Could you check a few things on this model? Use its own coordinates, in mm. Face numbers are marked on the shaded views. A direction names the side the tool comes from. Coordinates: 2 decimals unless noted, no trailing zeros. Order: outer loops, then holes, each group sorted by start corner. A loop starts at its lowest first (then second) coordinate and runs counter-clockwise, first axis right, second up. Notation, with made-up numbers: (26.5, -25) -> (83.5, -25) arc R30 ccw to (83.5, 4) -> close; hole circle Ø5 at (81.5, 52). An arc over 180 degrees is marked (long way). Return JSON: item names as keys, results as strings. Group by question number.
from build123d import *

# Parameters (mm, degrees)
EXTRUDE1_DEPTH                         = 25.4
EXTRUDE1_DEPTH_BACK                    = 50.8
SKETCH2_W                              = 119.38
SKETCH2_H                              = 22.225
EXTRUDE2_DEPTH                         = 3.175
SKETCH3_W                              = 3.175
SKETCH3_H                              = 22.225
EXTRUDE3_DEPTH                         = 19.05
TAP_DRILL_FOR_1_2_TAP1_D               = 11.50874
TAP_DRILL_FOR_1_2_TAP1_DEPTH           = 6.35
TAP_DRILL_FOR_1_2_TAP1_TIP             = 3.45757432
TAP_DRILL_FOR_1_2_TAP1_ON_FACE_2_D     = 11.50874
TAP_DRILL_FOR_1_2_TAP1_ON_FACE_2_DEPTH = 6.35
TAP_DRILL_FOR_1_2_TAP1_ON_FACE_2_TIP   = 3.45757432
F_8_CLEARANCE_HOLE1_D                  = 4.4958
F_8_CLEARANCE_HOLE1_DEPTH              = 6.35
F_8_CLEARANCE_HOLE1_TIP                = 1.350674586
F_8_CLEARANCE_HOLE1_ON_FACE_2_D        = 4.4958
F_8_CLEARANCE_HOLE1_ON_FACE_2_DEPTH    = 6.35
F_8_CLEARANCE_HOLE1_ON_FACE_2_TIP      = 1.350674586
FILLET1_R                              = 6.35
FILLET3_R                              = 3.175
SKETCH7_W                              = 81.28
SKETCH7_H                              = 3.175
EXTRUDE4_DEPTH                         = 25.4
FILLET4_R                              = 6.35
F_6_CLEARANCE_HOLE1_D                  = 3.7973
F_6_CLEARANCE_HOLE1_DEPTH              = 9.652
F_6_CLEARANCE_HOLE1_TIP                = 1.140824014
SKETCH8_W                              = 66.338719692
SKETCH8_H                              = 61.141500313
CUT_EXTRUDE1_DEPTH                     = 57.15


with BuildPart() as part:
    # Sketch1 → Extrude1 (new body, two sides)
    with BuildSketch(Plane(origin=(0, 0, 0), x_dir=(1, 0, 0), z_dir=(0, 1, 0))) as extrude1_sk:
        with BuildLine():
            Line((15.24, -11.1125), (-15.24, -11.1125))
            ThreePointArc((-15.24, -11.1125), (-19.730128061, -9.252628061), (-21.59, -4.7625))
            Line((-21.59, -4.7625), (-21.59, 4.7625))
            ThreePointArc((-21.59, 4.7625), (-19.730128061, 9.252628061), (-15.24, 11.1125))
            Line((-15.24, 11.1125), (15.24, 11.1125))
            ThreePointArc((15.24, 11.1125), (19.730128061, 9.252628061), (21.59, 4.7625))
            Line((21.59, 4.7625), (21.59, -4.7625))
            ThreePointArc((21.59, -4.7625), (19.730128061, -9.252628061), (15.24, -11.1125))
        make_face()
        with BuildLine():
            Line((-15.24, -7.9375), (-5.715, -7.9375))
            ThreePointArc((-5.715, -7.9375), (-3.46993597, -7.00756403), (-2.54, -4.7625))
            Line((-2.54, -4.7625), (-2.54, 4.7625))
            ThreePointArc((-2.54, 4.7625), (-3.46993597, 7.00756403), (-5.715, 7.9375))
            Line((-5.715, 7.9375), (-15.24, 7.9375))
            ThreePointArc((-15.24, 7.9375), (-17.48506403, 7.00756403), (-18.415, 4.7625))
            Line((-18.415, 4.7625), (-18.415, -4.7625))
            ThreePointArc((-18.415, -4.7625), (-17.48506403, -7.00756403), (-15.24, -7.9375))
        make_face(mode=Mode.SUBTRACT)
        with BuildLine():
            Line((15.24, 7.9375), (5.715, 7.9375))
            ThreePointArc((5.715, 7.9375), (3.46993597, 7.00756403), (2.54, 4.7625))
            Line((2.54, 4.7625), (2.54, -4.7625))
            ThreePointArc((2.54, -4.7625), (3.46993597, -7.00756403), (5.715, -7.9375))
            Line((5.715, -7.9375), (15.24, -7.9375))
            ThreePointArc((15.24, -7.9375), (17.48506403, -7.00756403), (18.415, -4.7625))
            Line((18.415, -4.7625), (18.415, 4.7625))
            ThreePointArc((18.415, 4.7625), (17.48506403, 7.00756403), (15.24, 7.9375))
        make_face(mode=Mode.SUBTRACT)
    extrude(amount=EXTRUDE1_DEPTH)
    extrude(extrude1_sk.sketch, amount=-EXTRUDE1_DEPTH_BACK)

    # Sketch2 → Extrude2 (add)
    with BuildSketch(Plane(origin=(0, 25.4, 0), x_dir=(-1, 0, 0), z_dir=(0, 1, 0))):
        Rectangle(SKETCH2_W, SKETCH2_H)
    extrude(amount=EXTRUDE2_DEPTH)

    # Sketch3 → Extrude3 (add)
    with BuildSketch(Plane.XZ.offset(-25.4)):
        with Locations((-58.1025, 0)):
            Rectangle(SKETCH3_W, SKETCH3_H)
        with Locations((58.1025, 0)):
            Rectangle(SKETCH3_W, SKETCH3_H)
    extrude(amount=EXTRUDE3_DEPTH)

    # Tap Drill for 1/2 Tap1
    with Locations(Plane(origin=(-59.69, 15.875, 0), x_dir=(0, 0, -1), z_dir=(-1, 0, 0))):
        with Locations((0, 0)):
            Hole(TAP_DRILL_FOR_1_2_TAP1_D / 2, depth=TAP_DRILL_FOR_1_2_TAP1_DEPTH)
            with Locations((0, 0, -(TAP_DRILL_FOR_1_2_TAP1_DEPTH + TAP_DRILL_FOR_1_2_TAP1_TIP / 2))):  # 118° drill point
                Cone(0, TAP_DRILL_FOR_1_2_TAP1_D / 2, TAP_DRILL_FOR_1_2_TAP1_TIP, mode=Mode.SUBTRACT)

    # Tap Drill for 1/2 Tap1 on face 2
    with Locations(Plane(origin=(59.69, 15.875, 0), x_dir=(0, 0, 1), z_dir=(1, 0, 0))):
        with Locations((0, 0)):
            Hole(TAP_DRILL_FOR_1_2_TAP1_ON_FACE_2_D / 2, depth=TAP_DRILL_FOR_1_2_TAP1_ON_FACE_2_DEPTH)
            with Locations((0, 0, -(TAP_DRILL_FOR_1_2_TAP1_ON_FACE_2_DEPTH + TAP_DRILL_FOR_1_2_TAP1_ON_FACE_2_TIP / 2))):  # 118° drill point
                Cone(0, TAP_DRILL_FOR_1_2_TAP1_ON_FACE_2_D / 2, TAP_DRILL_FOR_1_2_TAP1_ON_FACE_2_TIP, mode=Mode.SUBTRACT)

    # #8 Clearance Hole1
    with Locations(Plane(origin=(-21.59, 15.875, 0), x_dir=(0, 0, -1), z_dir=(-1, 0, 0))):
        with Locations((0, 0)):
            Hole(F_8_CLEARANCE_HOLE1_D / 2, depth=F_8_CLEARANCE_HOLE1_DEPTH)
            with Locations((0, 0, -(F_8_CLEARANCE_HOLE1_DEPTH + F_8_CLEARANCE_HOLE1_TIP / 2))):  # 118° drill point
                Cone(0, F_8_CLEARANCE_HOLE1_D / 2, F_8_CLEARANCE_HOLE1_TIP, mode=Mode.SUBTRACT)

    # #8 Clearance Hole1 on face 2
    with Locations(Plane(origin=(21.59, 15.875, 0), x_dir=(0, 0, 1), z_dir=(1, 0, 0))):
        with Locations((0, 0)):
            Hole(F_8_CLEARANCE_HOLE1_ON_FACE_2_D / 2, depth=F_8_CLEARANCE_HOLE1_ON_FACE_2_DEPTH)
            with Locations((0, 0, -(F_8_CLEARANCE_HOLE1_ON_FACE_2_DEPTH + F_8_CLEARANCE_HOLE1_ON_FACE_2_TIP / 2))):  # 118° drill point
                Cone(0, F_8_CLEARANCE_HOLE1_ON_FACE_2_D / 2, F_8_CLEARANCE_HOLE1_ON_FACE_2_TIP, mode=Mode.SUBTRACT)

    # Fillet1
    fillet1_edges = [part.edges().sort_by_distance(p)[0] for p in [
        (-58.1025, 6.35, -11.1125),
        (-58.1025, 6.35, 11.1125),
        (58.1025, 6.35, 11.1125),
        (58.1025, 6.35, -11.1125),
    ]]
    fillet(fillet1_edges, radius=FILLET1_R)

    # Fillet3
    fillet3_edges = [part.edges().sort_by_distance(p)[0] for p in [
        (-56.515, 25.4, 0),
        (56.515, 25.4, 0),
    ]]
    fillet(fillet3_edges, radius=FILLET3_R)

    # Sketch7 → Extrude4 (add)
    with BuildSketch(Plane.XY.offset(11.1125)):
        with Locations((0, 26.9875)):
            Rectangle(SKETCH7_W, SKETCH7_H)
    extrude(amount=EXTRUDE4_DEPTH)

    # Fillet4
    fillet4_edges = [part.edges().sort_by_distance(p)[0] for p in [
        (-40.64, 26.9875, 11.1125),
        (40.64, 26.9875, 11.1125),
    ]]
    fillet(fillet4_edges, radius=FILLET4_R)

    # #6 Clearance Hole1
    with Locations(Plane(origin=(31.75, 28.575, 26.9875), x_dir=(0, 0, 1), z_dir=(0, 1, 0))):
        with Locations((0, 0), (0, -63.5)):
            Hole(F_6_CLEARANCE_HOLE1_D / 2, depth=F_6_CLEARANCE_HOLE1_DEPTH)
            with Locations((0, 0, -(F_6_CLEARANCE_HOLE1_DEPTH + F_6_CLEARANCE_HOLE1_TIP / 2))):  # 118° drill point
                Cone(0, F_6_CLEARANCE_HOLE1_D / 2, F_6_CLEARANCE_HOLE1_TIP, mode=Mode.SUBTRACT)

    # Sketch8 → Cut-Extrude1 (cut)
    with BuildSketch(Plane.XZ.offset(50.8)):
        with Locations((-0.031295894, -3.796156427)):
            Rectangle(SKETCH8_W, SKETCH8_H)
    extrude(amount=-CUT_EXTRUDE1_DEPTH, mode=Mode.SUBTRACT)


solid = part.part
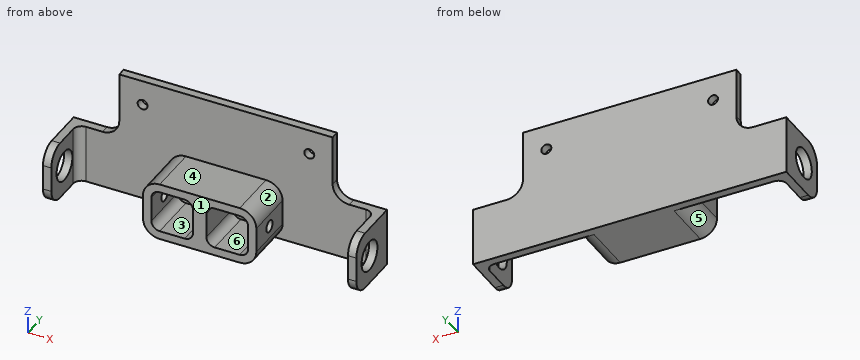
Q1. I'm going to push flat-ended pins straight in: pin 1 Ø10.5 at (x, y) = (8, 20) entering from +Z; pin 2 Ø6 at (x, z) = (39, 1) entering from -Y; pin 3 Ø1.5 at (x, y) = (21, 12) entering from -Z; pin 4 Ø2.5 at (x, z) = (-31.75, 26.99) entering from -Y. Where does each tip first touch, or does it pass through?
Q2. On a 3-axis mill with a long thin cutter (end or side, diameter ignored), from which of +Z, -Z, +X, -X, +Y, -Y can I reach the whole of each face in a straight line? I mean the marked faces 1, 2 and 3. Say none if no direction works.
Q3. I want a section at D-D on z = 30. Please give me the cut outline in (x, y) (3 decimals).
Q4. We'd pull the mould along Z, two halves only. Please class the marked faces 4, 5 and 6: pulls with the +Z half, pulls with the -Z half, needs draft (parallel to the pull), parting line crosses it, or undercut.
Q5. I want a section at A-A on x = -31.75. Please give me the cut outline in (y, z) (1 decimal).
Q6. I need wall thicknesses on line 1 along X through (y, z) = (10.75, 2.5) (3 decimals); line 2 along Y through (x, z) = (-20.9, 0) (3 decimals); line 3 along Z through (x, y) = (-8, 19.5). Which ranges of each line are inside material? Lowest first, please. Write a range as from..to.
Q7. I want a section at B-B on z = 0. State how many separate pieces and enclosed holes the cut face has, and give its area (3 significant figures).
Response values:
{
 "1": {"pin 1": "stops at z = 11.11", "pin 2": "stops at y = 25.4", "pin 3": "stops at z = -8.66", "pin 4": "passes through"},
 "2": {"face 1": "+Z, -Z, +X, -X, -Y", "face 2": "+Z, -Y", "face 3": "-Y"},
 "3": {"outline": "(-40.64, 25.4) -> (40.64, 25.4) -> (40.64, 28.575) -> (-40.64, 28.575) -> close"},
 "4": {"face 4": "pulls with the +Z half", "face 5": "pulls with the -Z half", "face 6": "undercut"},
 "5": {"outline": "(25.4, -11.1) -> (28.6, -11.1) -> (28.6, 25.1) -> (25.4, 25.1) -> close; (25.4, 28.9) -> (28.6, 28.9) -> (28.6, 36.5) -> (25.4, 36.5) -> close"},
 "6": {"line 1": "x = -21.59..-18.415, -2.54..2.54, 18.415..21.59", "line 2": "y = 6.35..13.627, 18.123..28.575", "line 3": "z = -11.11..-7.94, 7.94..11.11"},
 "7": {"separate pieces": "5", "enclosed holes": "0", "area": "620 mm²"}
}
